Geometry: final body of the model. Coordinates: model frame, mm. A direction names the side the tool comes from. Round coordinates to 2 decimals unless told otherwise and drop trailing zeros. Loops run counter-clockwise (first coordinate to the right, second up) from the corner with the lowest first, then second, coordinate; pieces in that order, holes last. Notation, with made-up numbers: (54.25, -14) - (106.25, -14) arc R6 ccw to (106.25, -9) - close; hole circle Ø9 at (-12.75, -19). An arc over 180 degrees is marked (long way). Answer as a JSON object with one key per item and string values. Group by question number.
Item 1: Line query: line 1 (Y direction, x = 15.5, z = 3); line 2 (Z direction, x = -16.5, y = 15); line 3 (X direction, y = 20.5, z = 3.05). Output: solid intervals per line, ascending.
Item 2: Section B-B (x = 26). Return the cut outline in (y, z), plus the area to 3 significant figures.
Item 3: Draft query along X for faces 1 (the face through (106.441, 2, 2)), 2 (the face through (94.942, 21.505, 2.028)), 3 (the face through (35, -22.061, 2)), 4 (the face through (-23.884, -19.025, 2.028)). Return one class per face: released by +X, released by -X, zero draft, split by the parting line, or undercut.
Item 4: First-contact query: pin 1 (3 mm diameter, centred on x = 39, y = -1.5, fed in from +Z). Flat tip, straight axial feed; report the tip coordinate or a pass-through.
Item 5: Section C-C (y = 1). Return the cut outline in (x, z).
Item 6: Section A-A (z = 3.3). Return the cut outline in (x, y).
Item 7: Reachability of faces 5 (the face through (35, 2, 2.61)), 6 (the face through (-23.884, 19.975, 2.028)) from +Z, -Z, +X, -X, +Y, -Y: full face, straight path, thin tool, end or side. Return the list, or none.
```python
from build123d import *

# Parameters (mm, degrees)
ESQUISSE1_W             = 140
ESQUISSE1_H             = 48
BOSS_EXTRU_1_DEPTH      = 4
ESQUISSE2_W             = 1.390122209
ESQUISSE2_H             = 30
ENL_V_MAT_EXTRU_1_DEPTH = 141
ESQUISSE4_R             = 1.5
ENL_V_MAT_EXTRU_3_DEPTH = 6


with BuildPart() as part:
    # Esquisse1 → Boss.-Extru.1 (new body)
    with BuildSketch(Plane.XY):
        with Locations((36.441041546, 1.939393939)):
            Rectangle(ESQUISSE1_W, ESQUISSE1_H)
    extrude(amount=BOSS_EXTRU_1_DEPTH)

    # Esquisse2 → Enlèv. mat.-Extru.1 (cut, through all)
    with BuildSketch(Plane.ZY.offset(33.558958454)):
        with Locations((3.304938896, 1.939393939)):
            Rectangle(ESQUISSE2_W, ESQUISSE2_H)
    extrude(amount=-ENL_V_MAT_EXTRU_1_DEPTH, mode=Mode.SUBTRACT)

    # Esquisse4 → Enlèv. mat.-Extru.3 (cut)
    with BuildSketch(Plane.XY.offset(4)):
        with Locations((-23.558958454, 21.439393939)):
            Circle(ESQUISSE4_R)
        with Locations((96.441041546, 21.439393939)):
            Circle(ESQUISSE4_R)
        with Locations((-23.558958454, -17.560606061)):
            Circle(ESQUISSE4_R)
        with Locations((96.441041546, -17.560606061)):
            Circle(ESQUISSE4_R)
    extrude(amount=-ENL_V_MAT_EXTRU_3_DEPTH, mode=Mode.SUBTRACT)


solid = part.part
```
Values:
{
 "1": {"line 1": "y = -22.06 to -13.06, 16.94 to 25.94", "line 2": "z = 0 to 2.61", "line 3": "x = -33.56 to -24.73, -22.39 to 95.27, 97.61 to 106.44"},
 "2": {"outline": "(-22.06, 0) - (25.94, 0) - (25.94, 4) - (16.94, 4) - (16.94, 2.61) - (-13.06, 2.61) - (-13.06, 4) - (-22.06, 4) - close", "area": "150 mm^2"},
 "3": {"face 1": "released by +X", "face 2": "undercut", "face 3": "zero draft", "face 4": "undercut"},
 "4": {"pin 1": "stops at z = 2.61"},
 "5": {"outline": "(-33.56, 0) - (106.44, 0) - (106.44, 2.61) - (-33.56, 2.61) - close"},
 "6": {"outline": "(-33.56, -22.06) - (106.44, -22.06) - (106.44, -13.06) - (-33.56, -13.06) - close; (-33.56, 16.94) - (106.44, 16.94) - (106.44, 25.94) - (-33.56, 25.94) - close; hole circle Ø3 at (-23.56, -17.56); hole circle Ø3 at (-23.56, 21.44); hole circle Ø3 at (96.44, -17.56); hole circle Ø3 at (96.44, 21.44)"},
 "7": {"face 5": "+Z, +X, -X", "face 6": "+Z, -Z"}
}
